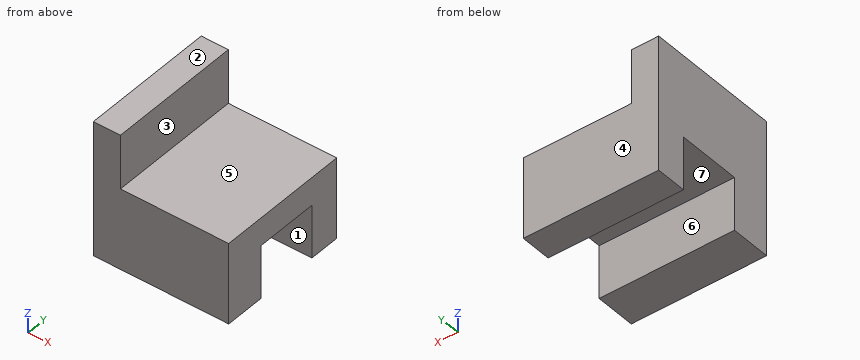
from build123d import *

# Parameters (mm, degrees)
F0_W     = 100
F0_H     = 100
F1_DEPTH = 100
F2_W     = 80
F2_H     = 100
F3_DEPTH = 40
F4_W     = 47.27444
F4_H     = 39.339293
F5_DEPTH = 100.001


with BuildPart() as f1:
    # F0 (on Top) → F1 (new body)
    with BuildSketch(Plane.XY):
        with Locations((-0.449351, 3.352783)):
            Rectangle(F0_W, F0_H)
    extrude(amount=F1_DEPTH)

    # F2 (on face) → F3 (cut)
    with BuildSketch(Plane.XY.offset(100)):
        with Locations((9.550649, 3.352783)):
            Rectangle(F2_W, F2_H)
    extrude(amount=-F3_DEPTH, mode=Mode.SUBTRACT)

    # F4 (on face) → F5 (cut, through all)
    with BuildSketch(Plane.YZ.offset(49.550649)):
        with Locations((6.754881, 19.669646)):
            Rectangle(F4_W, F4_H)
    extrude(amount=-F5_DEPTH, mode=Mode.SUBTRACT)


solid = f1.part
Work out the finished part from the listing and answer in its coordinate system (mm). Face numbers are marked on the shaded views. A direction names the side the tool comes from. Round coordinates to 2 decimals unless told otherwise and drop trailing zeros. Loops run counter-clockwise (first coordinate to the right, second up) from the corner with the lowest first, then second, coordinate; pieces in that order, holes last. Notation, with made-up numbers: M 41.5,-30 L 83.5,-30 A22 ccw 83.5,-7 Z; hole C 55,77 d9. An arc over 180 degrees is marked long. One line per question, with ' | ' between items. Start each with the question number.
(1) A cutting plane is placed at C-C on y = -24. Write down the section's boundary in (x, z).
(2) Find the intervals of material crossed by line 1 (Y direction, x = -28.5, z = 36.5); line 2 (Z direction, x = 18, y = -14); line 3 (Z direction, x = -30, y = 30.5), in increasing order.
(3) A cutting plane is placed at D-D on z = 87.5. Write down the section's boundary in (x, y), plus the area to 3 significant figures.
(4) A cutting plane is placed at A-A on z = 22. Write down the section's boundary in (x, y), plus the area to 3 significant figures.
(5) For a pull along Y with two mould halves and no side action, classify the marked faces 4, 5, 6 and 7 as released by +Y, released by -Y, zero draft, split by the parting line, or undercut.
(6) A cutting plane is placed at B-B on x = -36. Write down the section's boundary in (y, z), plus the area to 3 significant figures.
(7) Flat-ended cylindrical pins translate along their axes: pin 1 Ø8 at (y, z) = (-8, 36) entering from +X; pin 2 Ø12 at (y, z) = (-14, 72) entering from +X; pin 3 Ø12 at (x, y) = (27, 22) entering from -Z; pin 4 Ø24 at (x, y) = (28, 12) entering from +Z. Find the tip coordinate at first contact, or state that the pin passes through.
(8) A tool of negligible diameter and unlimited length cuts with its end or side. For the marked faces 1, 2 and 3, from which of +Z, -Z, +X, -X, +Y, -Y can it reach the whole face along a straight path? Write none if from no direction.
Geometry check:
1) outline: M -50.45,0 L 49.55,0 L 49.55,60 L -30.45,60 L -30.45,100 L -50.45,100 Z
2) line 1: y = -46.65 to -16.88, 30.39 to 53.35 | line 2: z = 39.34 to 60 | line 3: z = 0 to 60
3) outline: M -50.45,-46.65 L -30.45,-46.65 L -30.45,53.35 L -50.45,53.35 Z | area: 2,000 mm²
4) outline: M -50.45,-46.65 L 49.55,-46.65 L 49.55,-16.88 L -50.45,-16.88 Z; M -50.45,30.39 L 49.55,30.39 L 49.55,53.35 L -50.45,53.35 Z | area: 5,270 mm²
5) face 4: released by +Y | face 5: zero draft | face 6: undercut | face 7: undercut
6) outline: M -46.65,0 L -16.88,0 L -16.88,39.34 L 30.39,39.34 L 30.39,0 L 53.35,0 L 53.35,100 L -46.65,100 Z | area: 8,140 mm²
7) pin 1: stops at x = 49.55 | pin 2: stops at x = -30.45 | pin 3: stops at z = 39.34 | pin 4: stops at z = 60
8) face 1: -Z, +X, -X | face 2: +Z, +X, -X, +Y, -Y | face 3: +Z, +X, +Y, -Y
